Can you work these out from the model? Positions are in its coordinate system, mm. Face numbers are marked on the shaded views. A direction names the side the tool comes from. Coordinates: 2 decimals unless noted, no trailing zeros. Order: outer loops, then holes, each group sorted by start corner. A loop starts at its lowest first (then second) coordinate and runs counter-clockwise, first axis right, second up. Notation, with made-up numbers: (-14.5, 24.5) -> (43.5, 24.5) arc R21 cw to (43.5, 31.5) -> close; hole circle Ø11 at (10.5, 65.5). An arc over 180 degrees is marked (long way). Answer as CSV lines item,"result".
from build123d import *

# Parameters (mm, degrees)
F1_DEPTH = 33.782
F3_DEPTH = 11.0998


with BuildPart() as f1:
    # F0 (on Front) → F1 (new body)
    with BuildSketch(Plane.XZ):
        with BuildLine():
            Line((-60.427879, 66.98028), (-59.325351, 43.042825))
            ThreePointArc((-59.325351, 43.042825), (-47.907887, 55.562817), (-60.427879, 66.98028))
        make_face()
    extrude(amount=F1_DEPTH)

    # F2 (on face) → F3 (join)
    with BuildSketch(Plane.XZ.offset(33.782)):
        with BuildLine():
            Line((-60.208346, 62.213896), (-59.544884, 47.809209))
            ThreePointArc((-59.544884, 47.809209), (-52.674271, 55.343283), (-60.208346, 62.213896))
        make_face()
    extrude(amount=F3_DEPTH)


solid = f1.part
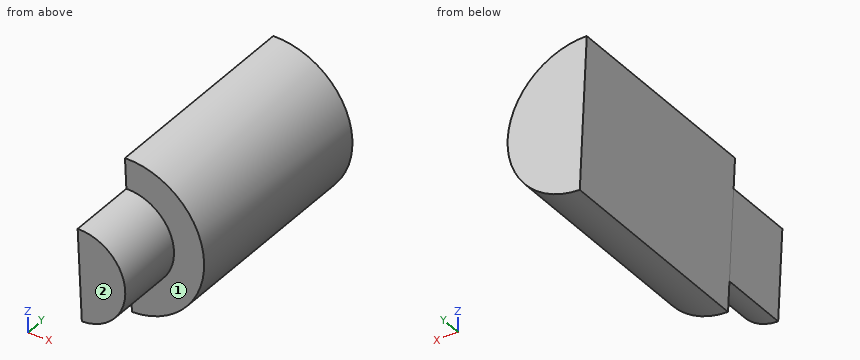
Q1. Imagine slicing it at D-D (x = -55.75). List the corners of the cut face in (y, z) for me.
Solution:
outline,"(-44.88, 49.1) -> (-33.78, 49.1) -> (-33.78, 43.76) -> (0, 43.76) -> (0, 66.26) -> (-33.78, 66.26) -> (-33.78, 60.92) -> (-44.88, 60.92) -> close"
Q2. Imagine slicing it at B-B (z = 58.5). List the corners of the cut face in (x, y) for me.
Solution:
outline,"(-60.04, -44.88) -> (-53.57, -44.88) -> (-53.57, -33.78) -> (-48.41, -33.78) -> (-48.41, 0) -> (-60.04, 0) -> close"
Q3. Imagine slicing it at A-A (x = -53.5). List the corners of the cut face in (y, z) for me.
Solution:
outline,"(-44.88, 51.65) -> (-33.78, 51.65) -> (-33.78, 44.87) -> (0, 44.87) -> (0, 65.16) -> (-33.78, 65.16) -> (-33.78, 58.38) -> (-44.88, 58.38) -> close"
Q4. Which directions (+Z, -Z, +X, -X, +Y, -Y) give clear straight access to the entire face, cutting with the end or side of a thin tool? Please do the marked faces 1 and 2.
Solution:
face 1,"+X, -Y"
face 2,"+Z, -Z, +X, -X, -Y"
Q5. If I drill on line 1 (Y direction, x = -55.5, z = 46.5); line 2 (Z direction, x = -55.5, y = -26.5) (3 decimals); line 3 (Z direction, x = -53.5, y = -31.5), over which ranges is the centre line in solid material (lowest first)?
Solution:
line 1,"-33.78 to 0"
line 2,"43.858 to 66.165"
line 3,"44.87 to 65.16"
Q6. Imagine slicing it at C-C (y = -32). List the corners of the cut face in (x, z) for me.
Solution:
outline,"(-60.43, 66.98) -> (-59.33, 43.04) arc R11.98 ccw to start"
Q7. For P1, Ø6, axis at x = -52.5, y = -30.5, coming from the -Z side; P2, Ø3, axis at x = -50, y = -22.5, coming from the -Z side; P3, Ø4, axis at y = -21, z = 54.5, coming from the -X side, each with a flat end and sliding along its axis, tell me the tip position at first contact or that it passes through.
Solution:
P1,"z = 43.86"
P2,"z = 46.44"
P3,"x = -59.95"
